Geometry: final body of the model. Coordinates: model frame, mm. A direction names the side the tool comes from. Give positions to 0.01 mm unless a question says otherwise; leave off trailing zeros. Loops run counter-clockwise (first coordinate to the right, second up) from the corner with the lowest first, then second, coordinate; pieces in that order, holes last. Notation, with made-up numbers: (50, 39) - (107, 39) arc R16 ccw to (107, 65) - close; hole circle Ø11 at (87, 34.25). An arc over 180 degrees is marked (long way). Use one line per item in the form item = value.
```python
from build123d import *

# Parameters (mm, degrees)
F0_W     = 153.613642
F0_H     = 149.788901
F1_DEPTH = 279.4
F2_R     = 66.386711
F3_DEPTH = 254


with BuildPart() as f1:
    # F0 (on Top) → F1 (new body)
    with BuildSketch(Plane.XY):
        with Locations((-1.47555, 1.547002)):
            Rectangle(F0_W, F0_H)
    extrude(amount=F1_DEPTH)

    # F2 (on face) → F3 (cut)
    with BuildSketch(Plane.XY.offset(279.4)):
        Circle(F2_R)
    extrude(amount=-F3_DEPTH, mode=Mode.SUBTRACT)


solid = f1.part
```
(1) Cut plane A-A (z = 160.5). Return the cut outline in (x, y).
Solution:
outline = (-78.28, -73.35) - (75.33, -73.35) - (75.33, 76.44) - (-78.28, 76.44) - close; hole circle Ø132.77 at (0, 0)
(2) Cut plane B-B (y = 0). Return the cut outline in (x, z), plus the area to 3 significant figures.
Solution:
outline = (-78.28, 0) - (75.33, 0) - (75.33, 279.4) - (66.39, 279.4) - (66.39, 25.4) - (-66.39, 25.4) - (-66.39, 279.4) - (-78.28, 279.4) - close
area = 9,200 mm2
(3) Pull-direction query (Y, two-part tool) for faces 3 (the face through (-3, 76.441, 138)), 4 (the face through (-1, 1, 25.4)), 5 (the face through (-3, 69, 279.4)); classes: released by +Y, released by -Y, zero draft, split by the parting line, or undercut.
Solution:
face_3 = released by +Y
face_4 = undercut
face_5 = zero draft
(4) Material intervals for L1, parallel to Y at x = 0, z = 149; L2, parallel to X at y = -50, z = 205; L3, parallel to X at y = -53, z = 122.5, sorted ascending. Write a range as from..to.
Solution:
L1 = -73.35..-66.39, 66.39..76.44
L2 = -78.28..-43.67, 43.67..75.33
L3 = -78.28..-39.98, 39.98..75.33
(5) Cut plane C-C (x = 28.5). Return the cut outline in (y, z), plus the area to 3 significant figures.
Solution:
outline = (-73.35, 0) - (76.44, 0) - (76.44, 279.4) - (59.96, 279.4) - (59.96, 25.4) - (-59.96, 25.4) - (-59.96, 279.4) - (-73.35, 279.4) - close
area = 11,400 mm2
(6) Access query for faces 1 (the face through (-78.282, 0, 138)), 2 (the face through (63.32, 19.94, 154.18)). Directions: +Z, -Z, +X, -X, +Y, -Y. A direction counts if a zero-diameter tool reaches every point of the face in a straight line with its end or side. Return the directions, or none.
Solution:
face_1 = +Z, -Z, -X, +Y, -Y
face_2 = +Z
